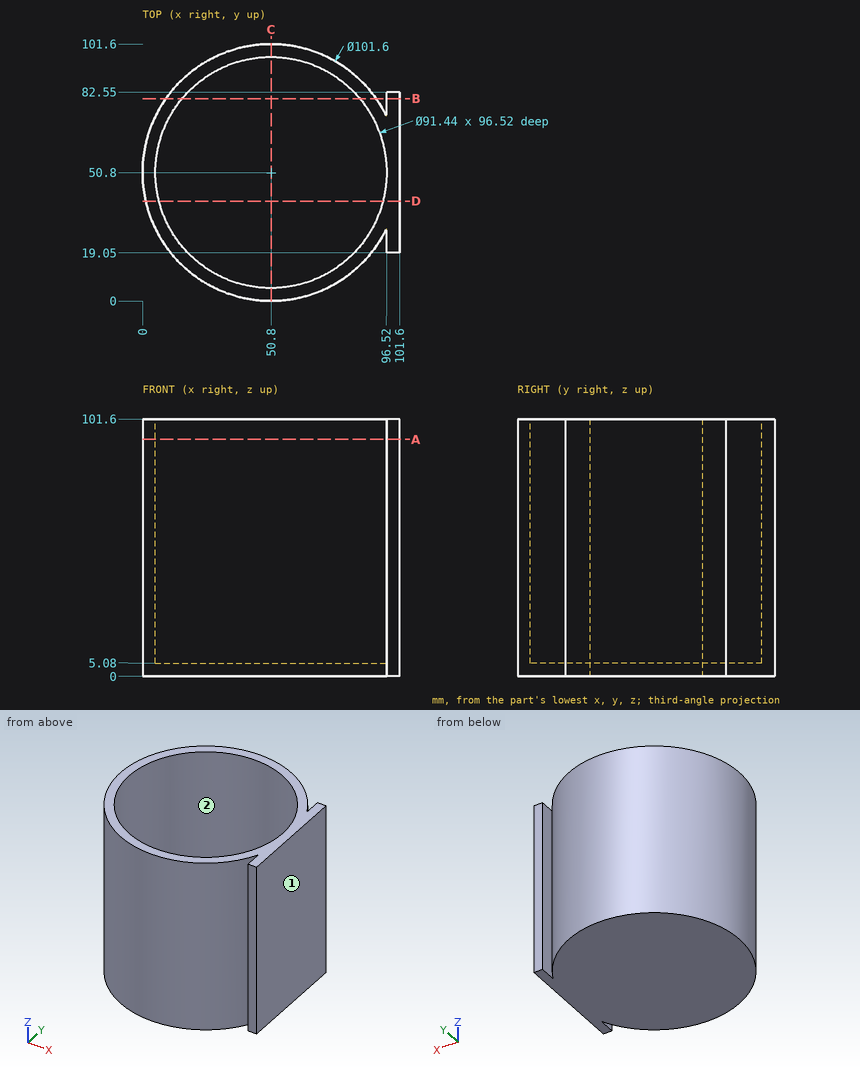
Study the drawing (mm; zero at the part's minimum x, y, z) and answer. Round coordinates to 2 decimals unless told otherwise and drop trailing zeros. Order: outer loops, then holes, each group sorted by start corner. A loop starts at its lowest first (then second) coordinate and runs counter-clockwise, first axis right, second up. Notation, with made-up numbers: (86, 50.25) -> (128, 50.25) arc R11 ccw to (128, 56.25) -> close; hole circle Ø8 at (-28.5, 68). An arc over 180 degrees is marked (long way). Write each question's results on one line, items separated by ' | '. Start each with the question number.
Q1. Straight lines are drawn through the part: probe 1 along Y at (x, z) = (50.8, 45); probe 2 along X at (y, z) = (74.5, 37.5); probe 3 along X at (y, z) = (80.5, 83.5). For each, find the intervals that lie inside material, in ascending order. Write a range as from..to.
Q2. Each of these flat-tipped pins is pushed along its axis until it touches: pin 1 (4 mm diameter, centred on y = 18, z = 28.5, fed in from +X); pin 2 (5.5 mm diameter, centred on x = 98.5, z = 63.5, fed in from -Y); pin 3 (10.5 mm diameter, centred on y = 79, z = 33.5, fed in from -X); pin 4 (1 mm diameter, centred on y = 33, z = 90.5, fed in from -X). Where does it stop, or does it pass through?
Q3. Find section C-C (x = 50.8). Determine the outline of the cut face in (y, z).
Q4. Find section D-D (y = 39.5). Determine the outline of the cut face in (x, z).
Q5. Find section B-B (y = 80). Determine the outline of the cut face in (x, z), then the cut area to 3 significant figures.
Q6. Find section A-A (z = 93.5). Determine the outline of the cut face in (x, y).
Q7. The mould has two halves that part along Y. Classify the marked faces 1 and 2: pulls with the +Y half, pulls with the -Y half, needs draft (parallel to the pull), parting line crosses it, or undercut.
Worked answers:
1) probe 1: y = 0..5.08, 96.52..101.6 | probe 2: x = 5.87..11.7, 89.9..95.73, 96.52..101.6 | probe 3: x = 9.59..16.04, 85.56..92.01, 96.52..101.6
2) pin 1: stops at x = 101.6 | pin 2: stops at y = 19.05 | pin 3: stops at x = 5.48 | pin 4: stops at x = 3.04
3) outline: (0, 0) -> (101.6, 0) -> (101.6, 101.6) -> (96.52, 101.6) -> (96.52, 5.08) -> (5.08, 5.08) -> (5.08, 101.6) -> (0, 101.6) -> close
4) outline: (1.27, 0) -> (101.6, 0) -> (101.6, 101.6) -> (95.1, 101.6) -> (95.1, 5.08) -> (6.5, 5.08) -> (6.5, 101.6) -> (1.27, 101.6) -> close
5) outline: (9.23, 0) -> (92.37, 0) -> (92.37, 101.6) -> (85.98, 101.6) -> (85.98, 5.08) -> (15.62, 5.08) -> (15.62, 101.6) -> (9.23, 101.6) -> close; (96.52, 0) -> (101.6, 0) -> (101.6, 101.6) -> (96.52, 101.6) -> close | area: 2,170 mm2
6) outline: (96.52, 19.05) -> (101.6, 19.05) -> (101.6, 82.55) -> (96.52, 82.55) -> (96.52, 72.94) arc R50.8 ccw (long way) to (96.52, 28.66) -> close; hole circle Ø91.44 at (50.8, 50.8)
7) face 1: needs draft | face 2: undercut
